Input: part model. Units: mm. Frame: model coordinates. Coordinates: 2 decimals unless noted, no trailing zeros. Write each loop counter-clockwise with the first axis right and the second up, starting at its lowest first coordinate (ties: lowest second). Pieces come first, ordered by that corner, then holes. Notation, with made-up numbers: M 68.25,-12.5 L 91.25,-12.5 A17 cw 91.25,14.5 Z; hole C 4,42.5 d7. An arc over 180 degrees is marked long. Answer as a JSON object with one key per item and string values. Group by question number.
from build123d import *

# Parameters (mm, degrees)
SKETCH1_R           = 17
BOSS_EXTRUDE1_DEPTH = 3.5
FILLET1_R           = 0.5


with BuildPart() as part:
    # Sketch1 → Boss-Extrude1 (new body)
    with BuildSketch(Plane(origin=(0, 0, 0), x_dir=(1, 0, 0), z_dir=(0, 1, 0))):
        Circle(SKETCH1_R)
        with BuildLine():
            Line((7.5, 17.7), (-7.5, 17.7))
            Line((-7.5, 17.7), (-9.5, 14.09787218))
            ThreePointArc((-9.5, 14.09787218), (0, 17), (9.5, 14.09787218))
            Line((9.5, 14.09787218), (7.5, 17.7))
        make_face()
    extrude(amount=BOSS_EXTRUDE1_DEPTH)

    # Fillet1
    fillet1_edges = [part.edges().sort_by_distance(p)[0] for p in [
        (0, 3.5, -17.7),
        (-8.5, 3.5, -15.89893609),
        (0, 3.5, 17),
        (-8.5, 0, -15.89893609),
        (0, 0, -17.7),
        (8.5, 0, -15.89893609),
        (0, 0, 17),
        (8.5, 3.5, -15.89893609),
        (-9.5, 1.75, -14.09787218),
        (-7.5, 1.75, -17.7),
        (7.5, 1.75, -17.7),
        (9.5, 1.75, -14.09787218),
    ]]
    fillet(fillet1_edges, radius=FILLET1_R)


solid = part.part
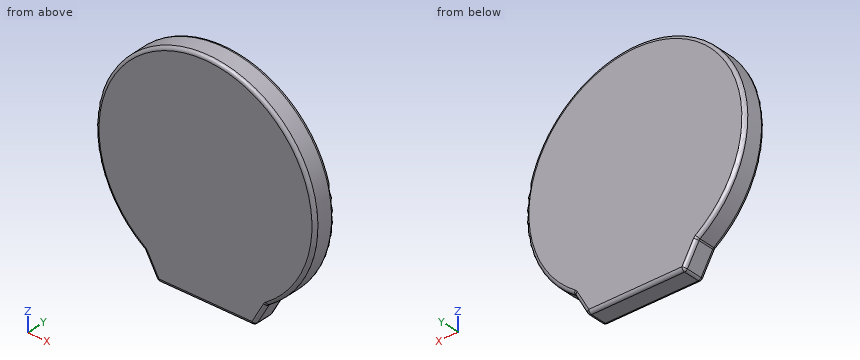
Q1. Section A-A, the plane y = 1.05. Return the cut outline in (x, z), and give its area (3 significant figures).
Q2. Pin query (flat end, axial travel): pin 1 Ø2 at (y, z) = (1.5, 1.5) entering from +X. Return the tip coordinate at first contact, or that it passes through.
Q3. Line query: line 1 (Z direction, x = 0.5, y = 1.5); line 2 (X direction, y = 2.75, z = -5); line 3 (Z direction, x = 8, y = 1). Output: solid intervals per line, ascending. Write a range as from..to.
Filled in:
{
 "1": {"outline": "M -9.6,-14.03 A0.5 cw -9.44,-14.2 L -7.64,-17.44 A0.5 ccw -7.21,-17.7 L 7.21,-17.7 A0.5 ccw 7.64,-17.44 L 9.44,-14.2 A0.5 cw 9.6,-14.03 A17 ccw long Z", "area": "932 mm^2"},
 "2": {"pin 1": "x = 16.99"},
 "3": {"line 1": "-17.7..16.99", "line 2": "-16.25..16.25", "line 3": "-16.8..15"}
}
